Part model, mm, in its own coordinate system. A direction names the side the tool comes from. Coordinates: 2 decimals unless noted, no trailing zeros. Loops run counter-clockwise (first coordinate to the right, second up) from the corner with the lowest first, then second, coordinate; pieces in that order, holes last. Notation, with made-up numbers: M -13.75,-40 L 25.25,-40 A19 cw 25.25,-22 Z; hole C -1.5,-31 d10. An arc over 180 degrees is marked long. Use CSV: the item, a comma, the result in double quotes. Start each with the question number.
from build123d import *

# Parameters (mm, degrees)
SALIENTE_EXTRUIR1_DEPTH = 3
CROQUIS2_W              = 3
CROQUIS2_H              = 15.2
SALIENTE_EXTRUIR2_DEPTH = 3
CROQUIS3_W              = 3
CROQUIS3_H              = 15.2
SALIENTE_EXTRUIR3_DEPTH = 3


with BuildPart() as part:
    # Croquis1 → Saliente-Extruir1 (new body)
    with BuildSketch(Plane.XY):
        with BuildLine():
            Line((134, -27.625), (70, -27.625))
            Line((70, -27.625), (70, -26.595))
            ThreePointArc((70, -26.595), (68.535533906, -23.059466094), (65, -21.595))
            Line((65, -21.595), (-65, -21.595))
            ThreePointArc((-65, -21.595), (-68.535533906, -23.059466094), (-70, -26.595))
            Line((-70, -26.595), (-70, -27.625))
            Line((-70, -27.625), (-134, -27.625))
            Line((-134, -27.625), (-134, -1.5))
            Line((-134, -1.5), (-131, -1.5))
            Line((-131, -1.5), (-131, -3))
            Line((-131, -3), (-128, -3))
            Line((-128, -3), (-128, 3))
            Line((-128, 3), (-131, 3))
            Line((-131, 3), (-131, 1.5))
            Line((-131, 1.5), (-134, 1.5))
            Line((-134, 1.5), (-134, 27.625))
            Line((-134, 27.625), (134, 27.625))
            Line((134, 27.625), (134, 1.5))
            Line((134, 1.5), (131, 1.5))
            Line((131, 1.5), (131, 3))
            Line((131, 3), (128, 3))
            Line((128, 3), (128, -3))
            Line((128, -3), (131, -3))
            Line((131, -3), (131, -1.5))
            Line((131, -1.5), (134, -1.5))
            Line((134, -1.5), (134, -27.625))
        make_face()
    extrude(amount=SALIENTE_EXTRUIR1_DEPTH)

    # Croquis2 → Saliente-Extruir2 (add)
    with BuildSketch(Plane(origin=(134, 0, 0), x_dir=(0, 0, -1), z_dir=(1, 0, 0))):
        with Locations((-1.5, 15.225)):
            Rectangle(CROQUIS2_W, CROQUIS2_H)
        with Locations((-1.5, -15.225)):
            Rectangle(CROQUIS2_W, CROQUIS2_H)
    extrude(amount=SALIENTE_EXTRUIR2_DEPTH)

    # Croquis3 → Saliente-Extruir3 (add)
    with BuildSketch(Plane.ZY.offset(134)):
        with Locations((1.5, 15.225)):
            Rectangle(CROQUIS3_W, CROQUIS3_H)
        with Locations((1.5, -15.225)):
            Rectangle(CROQUIS3_W, CROQUIS3_H)
    extrude(amount=SALIENTE_EXTRUIR3_DEPTH)


solid = part.part
1. Two-plate mould, pull along X, no slides. Class faces 1 (the face through (2, 0, 0)), 2 (the face through (68.574, -23.099, 1.479)): pulls with the +X half, pulls with the -X half, needs draft (parallel to the pull), parting line crosses it, or undercut.
2. Pin check, flat tips, straight feed: pin 1 (1.5 mm diameter, centred on y = -1, z = 1.5, fed in from -X); pin 2 (1.5 mm diameter, centred on y = 4, z = 0.5, fed in from +X); pin 3 (0.9 mm diameter, centred on x = -135.5, z = 2, fed in from -Y) (3 decimals). Stop position of each tip, or through.
3. Slice it at A-A, the plane x = -22. List the corners of the cut face in (y, z) (3 decimals), and give its area (3 significant figures).
4. Tool access for faces 3 (the face through (-68.496, -23.021, 1.479)), 4 (the face through (2, 0, 3)): list every direction of +Z, -Z, +X, -X, +Y, -Y with a clear straight run to the whole face (end or side of a thin tool).
5. Wall check: probe 1 along X at (y, z) = (6, 2.65); probe 2 along Y at (x, z) = (-10, 2.45) (3 decimals); probe 3 along X at (y, z) = (0.5, 0.35). Give the ranges that are in metal, low to high.
Found:
1,face 1,"needs draft"
1,face 2,"undercut"
2,pin 1,"x = -134"
2,pin 2,"x = 134"
2,pin 3,"y = -22.825"
3,outline,"M -21.595,0 L 27.625,0 L 27.625,3 L -21.595,3 Z"
3,area,"148 mm^2"
4,face 3,"+Z, -Z, -Y"
4,face 4,"+Z, +X, -X, +Y, -Y"
5,probe 1,"-134 to 134"
5,probe 2,"-21.595 to 27.625"
5,probe 3,"-128 to 128"
